The listing builds one solid part. Answer for the finished solid, in the listing's coordinates (mm). A direction names the side the tool comes from. Round coordinates to 2 decimals unless told otherwise and drop trailing zeros. Order: outer loops, then holes, each group sorted by start corner. A loop starts at its lowest first (then second) coordinate and runs counter-clockwise, first axis right, second up. Notation, with made-up numbers: (-31.75, -9.5) -> (26.25, -9.5) arc R16 cw to (26.25, 17.5) -> close; hole circle Ø11 at (71, 53). An arc over 180 degrees is marked (long way). Return JSON: item names as keys, results as strings. Group by question number.
(1) Determine the mould class of faces 3 (the face through (0.1, 33, 0.5)), 4 (the face through (-39, -38.5, 0.5)), 5 (the face through (39, 38.5, 0.5)), 6 (the face through (-1, 1, 1)) for opening direction Y: +Y half, -Y half, draft (parallel to the pull), parting line (faces both ways), or undercut.
(2) The part is cut by section C-C (z = 0.85). Determine the outline of the cut face in (x, y).
(3) Consider line 1 (Y direction, x = -8, z = 0.85); line 2 (Y direction, x = -47, z = 0.6); line 3 (Y direction, x = -3, z = 0.5). Determine where each line is inside the solid, lowest interval first. Write a range as [from, to].
(4) The part is cut by section D-D (x = 28). Determine the outline of the cut face in (y, z).
(5) The part is cut by section A-A (x = -10.5). Determine the outline of the cut face in (y, z).
(6) Which of the six approach directions +Z, -Z, +X, -X, +Y, -Y give full straight-line access (tool end or side, diameter ignored) to faces 1 (the face through (38.5, -39, 0.5)), 2 (the face through (-0.1, 41, 0.5))?
(7) The part is cut by section B-B (y = -37). Determine the outline of the cut face in (x, z).
from build123d import *

# Parameters (mm, degrees)
SKETCH1_R           = 2.5
SKETCH1_R_2         = 4
BOSS_EXTRUDE1_DEPTH = 1


with BuildPart() as part:
    # Sketch1 → Boss-Extrude1 (new body)
    with BuildSketch(Plane.XY):
        with BuildLine():
            Line((55, -21.257359313), (55, 21.257359313))
            ThreePointArc((55, 21.257359313), (54.771638598, 22.40540961), (54.121320344, 23.378679656))
            Line((54.121320344, 23.378679656), (23.378679656, 54.121320344))
            ThreePointArc((23.378679656, 54.121320344), (22.40540961, 54.771638598), (21.257359313, 55))
            Line((21.257359313, 55), (-52, 55))
            ThreePointArc((-52, 55), (-54.121320344, 54.121320344), (-55, 52))
            Line((-55, 52), (-55, -21.257359313))
            ThreePointArc((-55, -21.257359313), (-54.771638598, -22.40540961), (-54.121320344, -23.378679656))
            Line((-54.121320344, -23.378679656), (-23.378679656, -54.121320344))
            ThreePointArc((-23.378679656, -54.121320344), (-22.40540961, -54.771638598), (-21.257359313, -55))
            Line((-21.257359313, -55), (21.257359313, -55))
            ThreePointArc((21.257359313, -55), (22.40540961, -54.771638598), (23.378679656, -54.121320344))
            Line((23.378679656, -54.121320344), (54.121320344, -23.378679656))
            ThreePointArc((54.121320344, -23.378679656), (54.771638598, -22.40540961), (55, -21.257359313))
        make_face()
        with Locations((-47, 47)):
            Circle(SKETCH1_R, mode=Mode.SUBTRACT)
        with Locations((0, -37)):
            Circle(SKETCH1_R_2, mode=Mode.SUBTRACT)
        with BuildLine():
            Line((-25, 38), (-3.872983346, 38))
            ThreePointArc((-3.872983346, 38), (0, 41), (3.872983346, 38))
            Line((3.872983346, 38), (25, 38))
            ThreePointArc((25, 38), (26, 37), (25, 36))
            Line((25, 36), (3.872983346, 36))
            ThreePointArc((3.872983346, 36), (0, 33), (-3.872983346, 36))
            Line((-3.872983346, 36), (-25, 36))
            ThreePointArc((-25, 36), (-26, 37), (-25, 38))
        make_face(mode=Mode.SUBTRACT)
    extrude(amount=BOSS_EXTRUDE1_DEPTH)


solid = part.part
Answer below:
{
 "1": {"face 3": "undercut", "face 4": "-Y half", "face 5": "+Y half", "face 6": "draft"},
 "2": {"outline": "(-55, -21.26) arc R3 ccw to (-54.12, -23.38) -> (-23.38, -54.12) arc R3 ccw to (-21.26, -55) -> (21.26, -55) arc R3 ccw to (23.38, -54.12) -> (54.12, -23.38) arc R3 ccw to (55, -21.26) -> (55, 21.26) arc R3 ccw to (54.12, 23.38) -> (23.38, 54.12) arc R3 ccw to (21.26, 55) -> (-52, 55) arc R3 ccw to (-55, 52) -> close; hole circle Ø5 at (-47, 47); hole (-25, 36) -> (-3.87, 36) arc R4 ccw to (3.87, 36) -> (25, 36) arc R1 ccw to (25, 38) -> (3.87, 38) arc R4 ccw to (-3.87, 38) -> (-25, 38) arc R1 ccw to start; hole circle Ø8 at (0, -37)"},
 "3": {"line 1": "y = [-55, 36], [38, 55]", "line 2": "y = [-30.5, 44.5], [49.5, 55]", "line 3": "y = [-55, -39.65], [-34.35, 34.35], [39.65, 55]"},
 "4": {"outline": "(-49.5, 0) -> (49.5, 0) -> (49.5, 1) -> (-49.5, 1) -> close"},
 "5": {"outline": "(-55, 0) -> (36, 0) -> (36, 1) -> (-55, 1) -> close; (38, 0) -> (55, 0) -> (55, 1) -> (38, 1) -> close"},
 "6": {"face 1": "+Z, -Z, +X, -Y", "face 2": "+Z, -Z"},
 "7": {"outline": "(-40.5, 0) -> (-4, 0) -> (-4, 1) -> (-40.5, 1) -> close; (4, 0) -> (40.5, 0) -> (40.5, 1) -> (4, 1) -> close"}
}
